Autodesk Inventor part; units mm, degrees
ref_plane "YZ Plane" through (0, 0, 0) normal (1, 0, 0) x (0, 1, 0)
ref_plane "XZ Plane" through (0, 0, 0) normal (0, 1, 0) x (-1, 0, 0)
ref_plane "XY Plane" through (0, 0, 0) normal (0, 0, 1) x (1, 0, 0)
sketch "Sketch1" plane through (0, 0, 0) normal (0, 0, 1) x (1, 0, 0)
  line L0 (-25.4, -25.4) -> (25.4, -25.4)
  line L1 (25.4, -25.4) -> (25.4, 25.4)
  line L2 (25.4, 25.4) -> (-25.4, 25.4)
  line L3 (-25.4, 25.4) -> (-25.4, -25.4)
  line L4 (-25.4, -25.4) -> (25.4, 25.4) construction
  line L5 (25.4, -25.4) -> (-25.4, 25.4) construction
  point P0 (0, 0)
  dimension "d0" = 50.8
extrude "Extrusion1" add sketch "Sketch1" along normal mid plane 25.4
ref_plane "Work Plane1" through (0, 0, 9.525) normal (0, 0, 1) x (1, 0, 0)
sketch "Sketch2" plane through (0, 0, 9.525) normal (0, 0, 1) x (1, 0, 0)
  arc A0 (0, -6.6675) -> (0, 6.6675) centre (0, 0) ccw
  line L0 (0, -6.6675) -> (0, 6.6675)
  dimension "d5" = 6.6675
revolve "Revolution1" cut sketch "Sketch2" angle 360 about axis through (0, -6.6675, 9.525) along (0, 1, 0)
equation "\"d0\" = sideLength"
equation "\"d1\" = partDepth"
equation "\"d5\" = radiusofBallHole"
equation "\"d3\" = -workPlaneForBallDistanceFfromFontEdge"
equation "\"radiusofBallHole\" = 0.5 * diameterOfBallHole"
equation "\"sideLength\" = 50.8"
equation "\"partDepth\" = 25.4"
equation "\"workPlaneForBallDistanceFfromFontEdge\" = 3.175"
equation "\"allowancForBallToRotate\" = 0.635"
properties part number "socket"
Source: CAD feature listing. Evaluate the final solid. Frame: model axes, mm. Round coordinates to 2 decimals unless told otherwise and drop trailing zeros. Order: outer loops, then holes, each group sorted by start corner. A loop starts at its lowest first (then second) coordinate and runs counter-clockwise, first axis right, second up. Notation, with made-up numbers: (-11.75, -24.5) -> (47.25, -24.5) arc R12 cw to (47.25, -17.5) -> close; hole circle Ø2 at (82.5, 2). An arc over 180 degrees is marked (long way). Answer as CSV lines item,"result".
Item 1: Section B-B, the plane x = 15. Return loops of the section in (y, z).
A:
outline,"(-25.4, -12.7) -> (25.4, -12.7) -> (25.4, 12.7) -> (-25.4, 12.7) -> close"
Item 2: Section A-A, the plane z = 7.25. Return loops of the section in (x, y), plus the area to 3 significant figures.
A:
outline,"(-25.4, -25.4) -> (25.4, -25.4) -> (25.4, 25.4) -> (-25.4, 25.4) -> close; hole circle Ø12.53 at (0, 0)"
area,"2,460 mm²"
Item 3: Line query: L1, parallel to Z at x = -8, y = 7; L2, parallel to X at y = -3, z = 9.5; L3, parallel to Y at x = -5, z = 6. Output: solid intervals per line, ascending.
A:
L1,"-12.7 to 12.7"
L2,"-25.4 to -5.95, 5.95 to 25.4"
L3,"-25.4 to -2.65, 2.65 to 25.4"
Item 4: Pin query (flat end, axial travel): pin 1 Ø6 at (x, y) = (-18, 17) entering from +Z. Return the tip coordinate at first contact, or that it passes through.
A:
pin 1,"z = 12.7"
Item 5: Section D-D, the plane x = 5.5. Return loops of the section in (y, z) (3 decimals).
A:
outline,"(-25.4, -12.7) -> (25.4, -12.7) -> (25.4, 12.7) -> (2.031, 12.7) arc R3.769 cw (long way) to (-2.031, 12.7) -> (-25.4, 12.7) -> close"
